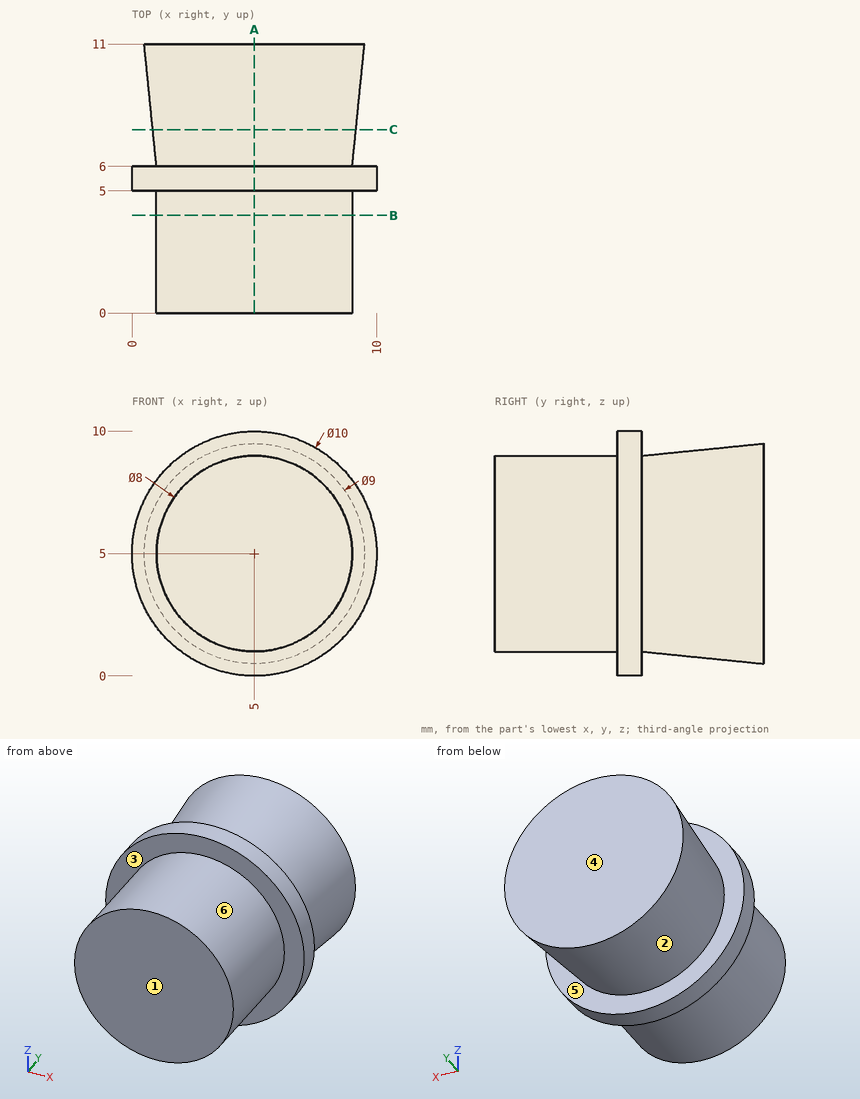
Geometry: see drawing. Coordinates: mm, zero at the bounding-box minimum. A direction names the side the tool comes from. Round coordinates to 2 decimals unless told otherwise and drop trailing zeros. Write each loop counter-clockwise with the first axis right and the second up, starting at its lowest first coordinate (ties: lowest second). Pieces come first, ordered by that corner, then holes.
1) Cut plane B-B (y = 4). Return the cut outline in (x, z).
2) Draft query along Y for the marked faces 4, 5 and 6. Return one class per face: pulls with the +Y half, pulls with the -Y half, needs draft (parallel to the pull), parting line crosses it, or undercut.
3) Reachability of the marked faces 1, 2 and 3 from +Z, -Z, +X, -X, +Y, -Y: full face, straight path, thin tool, end or side. Return the list, or none.
4) Contact query for flat-ended pins moving along their axis: P1, Ø3, axis at x = 4, y = 2, coming from the +Z side; P2, Ø1, axis at y = 5, z = 7.5, coming from the +X side. Output: stop coordinate, or through.
5) Ray query, L1, parallel to Y at x = 9.25, z = 6.75; L2, parallel to X at y = 0.5, z = 2.5; L3, parallel to Z at x = 3, y = 6.25. Return the intervals inside material, ascending.
6) Cut plane A-A (x = 5). Return the cut outline in (y, z), then the cut area to 3 significant figures.
7) Cut plane C-C (y = 7.5). Return the cut outline in (x, z).
Geometry says:
1. outline: circle Ø8 at (5, 5)
2. face 4: pulls with the +Y half
2. face 5: undercut
2. face 6: needs draft
3. face 1: +Z, -Z, +X, -X, -Y
3. face 2: none
3. face 3: -Y
4. P1: stops at z = 9
4. P2: stops at x = 9.58
5. L1: y = 5 to 6
5. L2: x = 1.88 to 8.12
5. L3: z = 1.51 to 8.49
6. outline: (0, 1) - (5, 1) - (5, 0) - (6, 0) - (6, 1) - (11, 0.5) - (11, 9.5) - (6, 9) - (6, 10) - (5, 10) - (5, 9) - (0, 9) - close
6. area: 92.5 mm2
7. outline: circle Ø8.3 at (5, 5)
